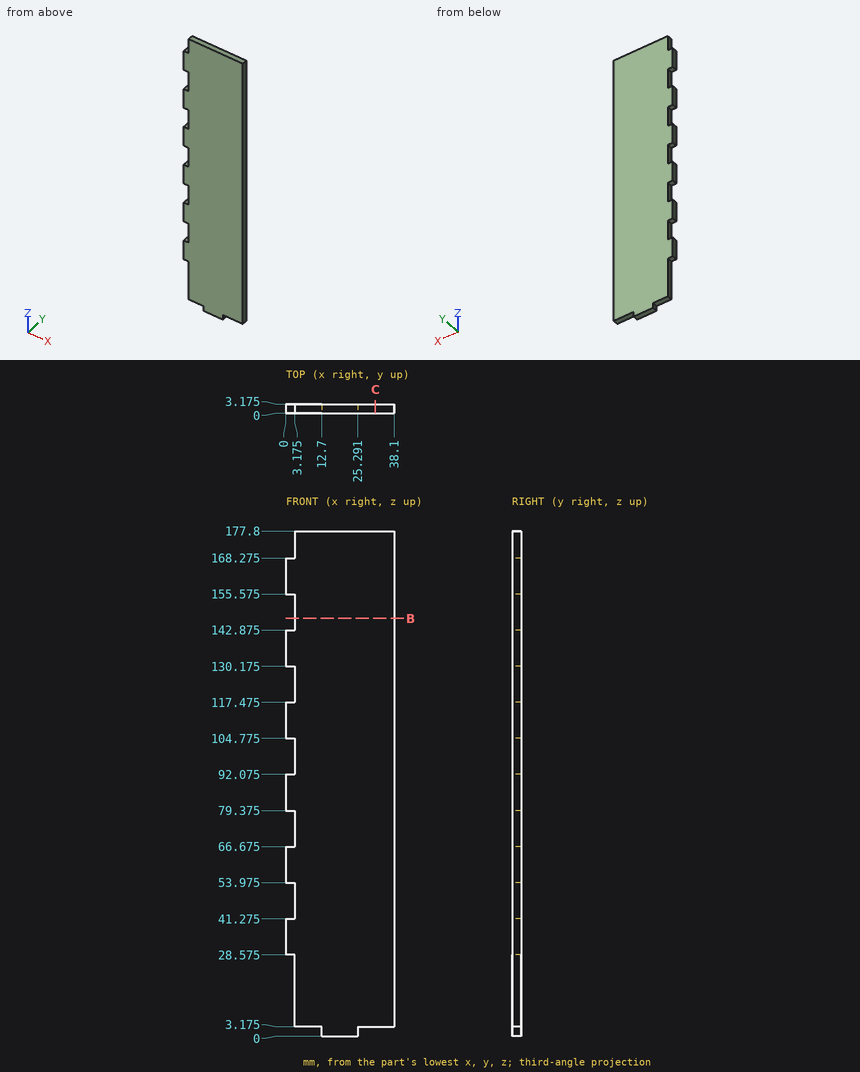
Drawing for the job (mm, zero at the part's lowest x, y, z). Round coordinates to 2 decimals unless told otherwise and drop trailing zeros. Write each loop counter-clockwise with the first axis right and the second up, starting at its lowest first coordinate (ties: lowest second). Pieces come first, ordered by that corner, then holes.
Item 1: Band-saw the part on C-C on x = 31.5. Write the cut outline in (y, z) (1 decimal).
Filled in:
outline: (0, 3.2) - (3.2, 3.2) - (3.2, 177.8) - (0, 177.8) - close
Item 2: Drop flat-ended pins along their axis: pin 1 Ø1 at (y, z) = (1, 73) entering from -X (3 decimals); pin 2 Ø1.6 at (x, y) = (33.5, 1.5) entering from -Z (3 decimals); pin 3 Ø1.6 at (x, y) = (2, 2) entering from +Z (3 decimals). Give the stop position or say it passes through.
Filled in:
pin 1: stops at x = 3.175
pin 2: stops at z = 3.175
pin 3: stops at z = 168.275
Item 3: Band-saw the part on B-B on z = 147. Write the cut outline in (x, y) (1 decimal).
Filled in:
outline: (3.2, 0) - (38.1, 0) - (38.1, 3.2) - (3.2, 3.2) - close
Item 4: Drill centre lines: L1, parallel to Z at x = 7, y = 0.25 (1 decimal); L2, parallel to X at y = 2.15, z = 47.5 (1 decimal). Where is each one in solid material? Low to high.
Filled in:
L1: z = 3.2 to 177.8
L2: x = 3.2 to 38.1
